CAD build for the part. Positions are in the model's coordinates, mm. Coordinates: 2 decimals unless noted, no trailing zeros. Write each loop counter-clockwise with the first axis right and the second up, starting at its lowest first coordinate (ties: lowest second). Pieces come first, ordered by that corner, then holes. Notation, with made-up numbers: (18.5, 74.25) - (71.5, 74.25) arc R31 ccw to (71.5, 105.25) - close; hole circle Ø1 at (30.25, 64). An arc over 180 degrees is marked (long way). One line per question, with ' | ' between items. Start each with the question number.
1. Probe line 1 (Y direction, x = 10, z = 1.2); line 2 (X direction, y = -10.5, z = 0.45); line 3 (Y direction, x = 11.5, z = 1.75). List the from-to ranges inside material, lowest first.
2. Band-saw the part on B-B, the plane x = 13.5. Write the cut outline in (y, z), then the cut area to 3 significant figures.
3. Band-saw the part on A-A, the plane x = 0.5. Give the number of separate pieces and of enclosed holes in the cut face, then the cut area to 3 significant figures.
4. Flat gauge pin, fed straight in: P1, Ø1.2, axis at x = -9.24, y = 3.83, coming from the +Z side. Where does the tip first touch, or does it go through?
from build123d import *

# Parameters (mm, degrees)
SKETCH1_R           = 16.71
SKETCH1_R_2         = 1
BOSS_EXTRUDE2_DEPTH = 2.21


with BuildPart() as part:
    # Sketch1 → Boss-Extrude2 (new body)
    with BuildSketch(Plane.XY):
        Circle(SKETCH1_R)
        Circle(SKETCH1_R_2, mode=Mode.SUBTRACT)
        with Locations((5, 0)):
            Circle(SKETCH1_R_2, mode=Mode.SUBTRACT)
        with Locations((10, 0)):
            Circle(SKETCH1_R_2, mode=Mode.SUBTRACT)
        with Locations((15, 0)):
            Circle(SKETCH1_R_2, mode=Mode.SUBTRACT)
        with Locations((3.535533906, -3.535533906)):
            Circle(SKETCH1_R_2, mode=Mode.SUBTRACT)
        with Locations((0, -5)):
            Circle(SKETCH1_R_2, mode=Mode.SUBTRACT)
        with Locations((-3.535533906, -3.535533906)):
            Circle(SKETCH1_R_2, mode=Mode.SUBTRACT)
        with Locations((-5, 0)):
            Circle(SKETCH1_R_2, mode=Mode.SUBTRACT)
        with Locations((-3.535533906, 3.535533906)):
            Circle(SKETCH1_R_2, mode=Mode.SUBTRACT)
        with Locations((0, 5)):
            Circle(SKETCH1_R_2, mode=Mode.SUBTRACT)
        with Locations((3.535533906, 3.535533906)):
            Circle(SKETCH1_R_2, mode=Mode.SUBTRACT)
        with Locations((9.238795325, -3.826834324)):
            Circle(SKETCH1_R_2, mode=Mode.SUBTRACT)
        with Locations((7.071067812, -7.071067812)):
            Circle(SKETCH1_R_2, mode=Mode.SUBTRACT)
        with Locations((3.826834324, -9.238795325)):
            Circle(SKETCH1_R_2, mode=Mode.SUBTRACT)
        with Locations((0, -10)):
            Circle(SKETCH1_R_2, mode=Mode.SUBTRACT)
        with Locations((-3.826834324, -9.238795325)):
            Circle(SKETCH1_R_2, mode=Mode.SUBTRACT)
        with Locations((-7.071067812, -7.071067812)):
            Circle(SKETCH1_R_2, mode=Mode.SUBTRACT)
        with Locations((-9.238795325, -3.826834324)):
            Circle(SKETCH1_R_2, mode=Mode.SUBTRACT)
        with Locations((-10, 0)):
            Circle(SKETCH1_R_2, mode=Mode.SUBTRACT)
        with Locations((-9.238795325, 3.826834324)):
            Circle(SKETCH1_R_2, mode=Mode.SUBTRACT)
        with Locations((-7.071067812, 7.071067812)):
            Circle(SKETCH1_R_2, mode=Mode.SUBTRACT)
        with Locations((-3.826834324, 9.238795325)):
            Circle(SKETCH1_R_2, mode=Mode.SUBTRACT)
        with Locations((0, 10)):
            Circle(SKETCH1_R_2, mode=Mode.SUBTRACT)
        with Locations((3.826834324, 9.238795325)):
            Circle(SKETCH1_R_2, mode=Mode.SUBTRACT)
        with Locations((7.071067812, 7.071067812)):
            Circle(SKETCH1_R_2, mode=Mode.SUBTRACT)
        with Locations((9.238795325, 3.826834324)):
            Circle(SKETCH1_R_2, mode=Mode.SUBTRACT)
        with Locations((13.858192988, -5.740251485)):
            Circle(SKETCH1_R_2, mode=Mode.SUBTRACT)
        with Locations((10.606601718, -10.606601718)):
            Circle(SKETCH1_R_2, mode=Mode.SUBTRACT)
        with Locations((5.740251485, -13.858192988)):
            Circle(SKETCH1_R_2, mode=Mode.SUBTRACT)
        with Locations((0, -15)):
            Circle(SKETCH1_R_2, mode=Mode.SUBTRACT)
        with Locations((-5.740251485, -13.858192988)):
            Circle(SKETCH1_R_2, mode=Mode.SUBTRACT)
        with Locations((-10.606601718, -10.606601718)):
            Circle(SKETCH1_R_2, mode=Mode.SUBTRACT)
        with Locations((-13.858192988, -5.740251485)):
            Circle(SKETCH1_R_2, mode=Mode.SUBTRACT)
        with Locations((-15, 0)):
            Circle(SKETCH1_R_2, mode=Mode.SUBTRACT)
        with Locations((-13.858192988, 5.740251485)):
            Circle(SKETCH1_R_2, mode=Mode.SUBTRACT)
        with Locations((-10.606601718, 10.606601718)):
            Circle(SKETCH1_R_2, mode=Mode.SUBTRACT)
        with Locations((-5.740251485, 13.858192988)):
            Circle(SKETCH1_R_2, mode=Mode.SUBTRACT)
        with Locations((0, 15)):
            Circle(SKETCH1_R_2, mode=Mode.SUBTRACT)
        with Locations((5.740251485, 13.858192988)):
            Circle(SKETCH1_R_2, mode=Mode.SUBTRACT)
        with Locations((10.606601718, 10.606601718)):
            Circle(SKETCH1_R_2, mode=Mode.SUBTRACT)
        with Locations((13.858192988, 5.740251485)):
            Circle(SKETCH1_R_2, mode=Mode.SUBTRACT)
    extrude(amount=BOSS_EXTRUDE2_DEPTH)


solid = part.part
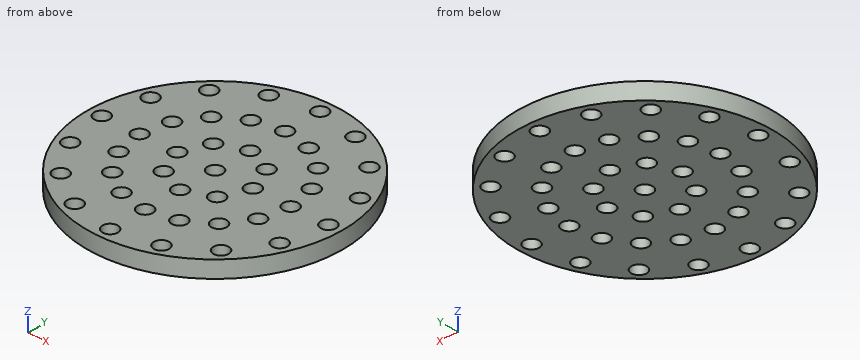
Filled in:
1) line 1: y = -13.39 to -11.4, -9.81 to -4.48, -3.18 to -1, 1 to 3.18, 4.48 to 9.81, 11.4 to 13.39 | line 2: x = -13 to -11.6, -9.61 to -0.87, 0.87 to 9.61, 11.6 to 13 | line 3: y = -12.12 to -11.06, -10.16 to 10.16, 11.06 to 12.12
2) outline: (-9.85, 0) - (-6.67, 0) - (-6.67, 2.21) - (-9.85, 2.21) - close; (-4.81, 0) - (4.81, 0) - (4.81, 2.21) - (-4.81, 2.21) - close; (6.67, 0) - (9.85, 0) - (9.85, 2.21) - (6.67, 2.21) - close | area: 35.3 mm²
3) separate pieces: 8 | enclosed holes: 0 | area: 47.0 mm²
4) P1: passes through
